Autodesk Inventor part; units mm, degrees
ref_plane "YZ Plane" through (0, 0, 0) normal (1, 0, 0) x (0, 1, 0)
ref_plane "XZ Plane" through (0, 0, 0) normal (0, 1, 0) x (-1, 0, 0)
ref_plane "XY Plane" through (0, 0, 0) normal (0, 0, 1) x (1, 0, 0)
sketch "Sketch1" plane through (0, 0, 0) normal (0, 0, 1) x (1, 0, 0)
  circle A0 centre (0, 0) radius 4.7625
  line L0 (12.7, -419.1) -> (12.7, 38.1)
  line L1 (12.7, 38.1) -> (-12.7, 38.1)
  line L2 (-12.7, 38.1) -> (-12.7, -419.1)
  line L3 (-12.7, -419.1) -> (12.7, -419.1)
  dimension "d0" = 9.525
  dimension "d2" = 12.7
  dimension "d3" = 38.1
  dimension "d4" = 457.2
extrude "Extrusion1" add sketch "Sketch1" along normal blind 25.4
sketch "Sketch2" plane through (0, 0, 25.4) normal (0, 0, 1) x (1, 0, 0)
  line L0 (12.7, -419.1) -> (-12.7, -419.1)
  line L1 (12.7, 38.1) -> (12.7, -419.1)
  circle A0 centre (0, -406.4) radius 3.175
  dimension "d7" = 12.7
  dimension "d8" = 12.7
  dimension "d9" = 6.35
extrude "Extrusion2" cut sketch "Sketch2" against normal up to next
properties part number "Stinger"
The model under review builds one solid part; all positions refer to its coordinate system, in mm. Coordinates: 2 decimals unless noted, no trailing zeros. Write each loop counter-clockwise with the first axis right and the second up, starting at its lowest first coordinate (ties: lowest second). Pieces come first, ordered by that corner, then holes. Notation, with made-up numbers: (11, -8.75) - (33, -8.75) arc R21 ccw to (33, 12.25) - close; hole circle Ø7 at (27.5, 67). An arc over 180 degrees is marked (long way). Answer in a Markdown table with one row per item. Add a question column.
Q1. Draft analysis for pull direction X (two halves, no side actions). For faces 1 (the face through (-3.78, 2.9, 12.52)), 2 (the face through (0, -419.1, 13)), 3 (the face through (-12.7, -187, 13)), 4 (the face through (12.7, -194, 13)), state which applies: +X half, -X half, draft (parallel to the pull), parting line (faces both ways), or undercut.
Q2. Consider section A-A on y = 0. Give the boundary of the cut face in (x, z).
Q3. Clearance check with a flat-ended pin moving along its axis: pin 1 (5.5 mm diameter, centred on x = 0, y = -406.4, fed in from -Z). State where the tip first meets the part, or that it passes through.
Q4. To check wall thickness, follow line 1 along Y through (x, z) = (0, 16.75) (1 decimal); line 2 along X through (y, z) = (-406.4, 15.5) (3 decimals); line 3 along Y through (x, z) = (2, 19). State the ranges of each line that lie inside material, in increasing order. Write a range as from..to.
Answers below:
| question | item | result |
|---|---|---|
| 1 | face 1 | undercut |
| 1 | face 2 | draft |
| 1 | face 3 | -X half |
| 1 | face 4 | +X half |
| 2 | outline | (-12.7, 0) - (-4.76, 0) - (-4.76, 25.4) - (-12.7, 25.4) - close; (4.76, 0) - (12.7, 0) - (12.7, 25.4) - (4.76, 25.4) - close |
| 3 | pin 1 | through |
| 4 | line 1 | -419.1..-409.6, -403.2..-4.8, 4.8..38.1 |
| 4 | line 2 | -12.7..-3.175, 3.175..12.7 |
| 4 | line 3 | -419.1..-408.87, -403.93..-4.32, 4.32..38.1 |
